Input: part model. Units: mm. Frame: model coordinates. Face numbers are marked on the shaded views. A direction names the side the tool comes from. Give positions to 0.01 mm unless a question says otherwise; leave off trailing zeros. Write each loop counter-clockwise with the first axis right and the second up, starting at its lowest first coordinate (ties: lowest second). Pieces come first, ordered by that corner, then holes. Notation, with made-up numbers: M 36.25,22.5 L 61.25,22.5 A27 cw 61.25,54.5 Z; hole C -14,10.25 d2. An arc over 180 degrees is marked long. Use CSV: the item, a comma, the result in double quotes. Start each with the question number.
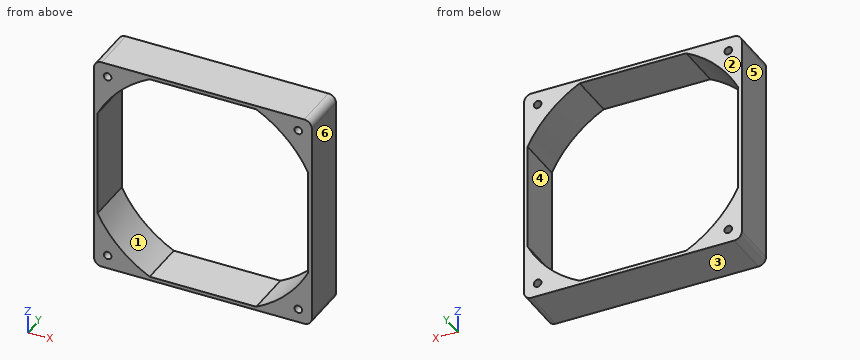
Autodesk Inventor part; units mm, degrees
ref_plane "YZ Plane" through (0, 0, 0) normal (1, 0, 0) x (0, 1, 0)
ref_plane "XZ Plane" through (0, 0, 0) normal (0, 1, 0) x (-1, 0, 0)
ref_plane "XY Plane" through (0, 0, 0) normal (0, 0, 1) x (1, 0, 0)
sketch "Sketch1" plane through (0, 0, 0) normal (0, 1, 0) x (-1, 0, 0)
  line L0 (0, 0) -> (120, 0)
  line L1 (120, 0) -> (120, -120)
  line L2 (120, -120) -> (0, -120)
  line L3 (0, -120) -> (0, 0)
  line L4 (112.5, -7.5) -> (7.5, -7.5) construction
  line L5 (7.5, -7.5) -> (7.5, -112.5) construction
  line L6 (7.5, -112.5) -> (112.5, -112.5) construction
  line L7 (112.5, -112.5) -> (112.5, -7.5) construction
  line L8 (112.5, -60) -> (120, -60) construction
  line L9 (60, -112.5) -> (60, -120) construction
  circle A0 centre (112.5, -7.5) radius 2.1167
  circle A1 centre (112.5, -112.5) radius 2.1167
  circle A2 centre (7.5, -112.5) radius 2.1167
  circle A3 centre (7.5, -7.5) radius 2.1167
  circle A4 centre (60, -60) radius 65
  line L10 (89.3428, -2) -> (30.6572, -2)
  line L11 (118, -30.6572) -> (118, -89.3428)
  line L12 (89.3428, -118) -> (30.6572, -118)
  line L13 (2, -30.6572) -> (2, -89.3428)
  point P0 (116.25, -60)
  point P1 (60, -116.25)
  dimension "d3" = 130
  dimension "d0" = 120
  dimension "d1" = 105
  dimension "d2" = 4.2333
  dimension "d4" = 2
extrude "Extrusion1" add sketch "Sketch1" along normal blind 26 contours L0 A4 L3 | L0 A4 L10 | A4 L13 L3 | L0 L1 A4 | A4 L2 L3 | L1 A4 L11 | A4 L12 L2 | L1 L2 A4
fillet "Fillet1" radius 4.2333 4 edges at (0, 13, -120) (-120, 13, -120) (-120, 13, 0) (0, 13, 0)
properties part number "120mm_fan"
Q1. Section C-C, the plane y = 15.5. Return the cut outline in (x, z), and give its area (3 significant figures).
Q2. Pull-direction query (X, two-part tool) for the marked faces 3, 4, 5 and 6; classes: released by +X, released by -X, zero draft, split by the parting line, or undercut.
Q3. Section A-A, the plane x = -66.5. Return the cut outline in (y, z), and give its area (3 significant figures).
Q4. Section B-B, the plane z = -33.5. Return the cut outline in (x, y), and give its area (3 significant figures).
Q5. Set-up query: the marked faces 1 and 2. Return all of +Z, -Z, +X, -X, +Y, -Y with unobstructed straight access to the full face (end or side cutting, diameter ignored); none if empty.
Q6. Material intervals for L1, parallel to Z at x = -53, y = 4.5; L2, parallel to Z at x = -112.5, y = 14.75, sorted ascending. Write a range as [from, to].
Q7. Section D-D, the plane z = -7.5. Return the cut outline in (x, y).
Check result:
1,outline,"M -120,-115.77 A4.23 ccw -115.77,-120 L -4.23,-120 A4.23 ccw 0,-115.77 L 0,-4.23 A4.23 ccw -4.23,0 L -115.77,0 A4.23 ccw -120,-4.23 Z; hole M -118,-89.34 A65 ccw -89.34,-118 L -30.66,-118 A65 ccw -2,-89.34 L -2,-30.66 A65 ccw -30.66,-2 L -89.34,-2 A65 ccw -118,-30.66 Z; hole C -112.5,-112.5 d4.23; hole C -112.5,-7.5 d4.23; hole C -7.5,-112.5 d4.23; hole C -7.5,-7.5 d4.23"
1,area,"2,160 mm²"
2,face 3,"zero draft"
2,face 4,"undercut"
2,face 5,"released by -X"
2,face 6,"released by +X"
3,outline,"M 0,-120 L 26,-120 L 26,-118 L 0,-118 Z; M 0,-2 L 26,-2 L 26,0 L 0,0 Z"
3,area,"104 mm²"
4,outline,"M -120,0 L -118,0 L -118,26 L -120,26 Z; M -2,0 L 0,0 L 0,26 L -2,26 Z"
4,area,"104 mm²"
5,face 1,"+Y, -Y"
5,face 2,"+Z, -Z, +X, -X, +Y"
6,L1,"z = [-120, -118], [-2, 0]"
6,L2,"z = [-120, -114.62], [-110.38, -98.32], [-21.68, -9.62], [-5.38, 0]"
7,outline,"M -120,0 L -114.62,0 L -114.62,26 L -120,26 Z; M -110.38,0 L -98.32,0 L -98.32,26 L -110.38,26 Z; M -21.68,0 L -9.62,0 L -9.62,26 L -21.68,26 Z; M -5.38,0 L 0,0 L 0,26 L -5.38,26 Z"
